from build123d import *

# Parameters (mm, degrees)
BOSS_EXTRUDE1_DEPTH = 10


with BuildPart() as part:
    # Sketch1 → Boss-Extrude1 (new body)
    with BuildSketch(Plane(origin=(0, 0, 0), x_dir=(1, 0, 0), z_dir=(0, 1, 0))):
        with BuildLine():
            Line((58.533362025, 10), (-60.218804352, 14.948006932))
            ThreePointArc((-60.218804352, 14.948006932), (-50.427672798, 10.155847962), (-46.466637975, 0))
            ThreePointArc((-46.466637975, 0), (-50.427672798, -10.155847962), (-60.218804352, -14.948006932))
            Line((-60.218804352, -14.948006932), (58.533362025, -10))
            ThreePointArc((58.533362025, -10), (48.533362025, 0), (58.533362025, 10))
        make_face()
        with BuildLine():
            Line((-61.466637975, -15), (-61.466637975, 15))
            ThreePointArc((-61.466637975, 15), (-76.466637975, 0), (-61.466637975, -15))
        make_face()
        with BuildLine():
            ThreePointArc((68.533362025, 0), (65.604429837, 7.071067812), (58.533362025, 10))
            Line((58.533362025, 10), (58.533362025, -10))
            ThreePointArc((58.533362025, -10), (65.604429837, -7.071067812), (68.533362025, 0))
        make_face()
        with BuildLine():
            Line((58.533362025, -10), (58.533362025, 10))
            ThreePointArc((58.533362025, 10), (48.533362025, 0), (58.533362025, -10))
        make_face()
        with BuildLine():
            Line((-60.218804352, 14.948006932), (-61.466637975, 15))
            Line((-61.466637975, 15), (-61.466637975, -15))
            Line((-61.466637975, -15), (-60.218804352, -14.948006932))
            ThreePointArc((-60.218804352, -14.948006932), (-50.427672798, -10.155847962), (-46.466637975, 0))
            ThreePointArc((-46.466637975, 0), (-50.427672798, 10.155847962), (-60.218804352, 14.948006932))
        make_face()
    extrude(amount=BOSS_EXTRUDE1_DEPTH)


solid = part.part
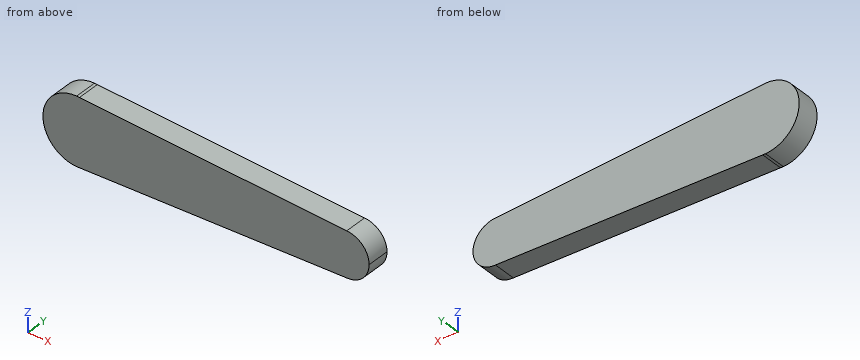
Part model, mm, in its own coordinate system. Coordinates: 2 decimals unless noted, no trailing zeros. Loops run counter-clockwise (first coordinate to the right, second up) from the corner with the lowest first, then second, coordinate; pieces in that order, holes last. Notation, with made-up numbers: (58.25, 79) - (100.25, 79) arc R18 ccw to (100.25, 86) - close; hole circle Ø8 at (35.25, 72.25). An arc over 180 degrees is marked (long way). Write each question's results on one line, items separated by ' | '. Start each with the question number.
Q1. Drop flat-ended pins along their axis: pin 1 Ø1 at (y, z) = (2, -4.5) entering from +X; pin 2 Ø3 at (x, y) = (-18.5, 7.5) entering from +Z; pin 3 Ø4 at (y, z) = (2.5, 9) entering from -X. Give the stop position or say it passes through.
Q2. Slice it at C-C on z = -8.5. Give the cut face in (x, y).
Q3. Slice it at B-B on x = 48.5. Give the cut face in (y, z), and give its area (3 significant figures).
Q4. Probe line 1 along X through (y, z) = (3.75, 0.5); line 2 along X through (y, z) = (0.5, -8.75); line 3 along Z through (x, y) = (-23.5, 2.5). List the from-to ranges inside material, lowest first.
Q5. Slice it at A-A on y = 2.5. Give the cut face in (x, z).
Answer:
1) pin 1: stops at x = 67.7 | pin 2: stops at z = 13.27 | pin 3: stops at x = -74.73
2) outline: (-73.83, 0) - (63.8, 0) - (63.8, 10) - (-73.83, 10) - close
3) outline: (0, -10.42) - (10, -10.42) - (10, 10.42) - (0, 10.42) - close | area: 208 mm2
4) line 1: x = -76.46 to 68.52 | line 2: x = -73.65 to 63.37 | line 3: z = -13.42 to 13.42
5) outline: (-61.47, -15) - (58.53, -10) arc R10 ccw to (58.53, 10) - (-61.47, 15) arc R15 ccw to start
